Autodesk Inventor part; units mm, degrees
ref_plane "Work Plane2" through (11.25, 70.4, 1) normal (0, 1, 0) x (0, 0, 1)
ref_plane "Work Plane3" through (11.25, 42.7, 1) normal (0, -1, 0) x (1, 0, 0)
ref_plane "Work Plane4" through (11.925, 37.7, 1.675) normal (0, -1, 0) x (1, 0, 0)
ref_plane "Work Plane1" through (25.625, 84.2, 15.375) normal (0, 1, 0) x (0, 0, -1)
sketch "Sketch1" plane through (25.625, 84.2, 15.375) normal (0, 1, 0) x (0, 0, -1)
  line L0 (11.5, -1.5) -> (11, -1.5)
  line L1 (11, -1.5) -> (11, 1.5)
  line L2 (11, 1.5) -> (11.5, 1.5)
  line L3 (11.5, 1.5) -> (11.5, -1.5)
  line L4 (-12, -1.5) -> (-12, 1.5)
  line L5 (-12, 1.5) -> (-11.5, 1.5)
  line L6 (-11.5, 1.5) -> (-11.5, -1.5)
  line L7 (-11.5, -1.5) -> (-12, -1.5)
  circle A0 centre (0, 0) radius 5
  circle A1 centre (0, 0) radius 13.7
  line L8 (18.875, -15.375) -> (18.875, 116.625)
  line L9 (18.875, 116.625) -> (15.375, 116.625)
  line L10 (15.375, -15.375) -> (15.375, 116.625)
  line L11 (18.875, -15.375) -> (15.375, -15.375)
  line L12 (15.375, -15.375) -> (0, -15.375)
  line L13 (0, -15.375) -> (0, 15.375)
  line L14 (0, 15.375) -> (15.375, 15.375)
  line L15 (15.375, 15.375) -> (15.375, -15.375)
  circle A2 centre (12.125, 12.125) radius 3.25
  circle A3 centre (12.125, -12.125) radius 3.25
  line L16 (8.875, 15.375) -> (8.875, 10.4367)
  point P0 (15.375, 25.625)
  point P1 (0, -13.7)
  dimension "d2" = 15.375
  dimension "d3" = 15.375
  dimension "d4" = 6.5
  dimension "d5" = 6.5
ref_plane "Work Plane2" through (11.25, 70.4, 1) normal (0, 1, 0) x (0, 0, 1)
extrude "Extrusion1" add sketch "Sketch1" along normal blind 4 and the other way blind 13.8 contours A1 L16 A2 L10 A3 L12 L13 | L16 L14 A2 | A2 | A3 L10 L12 | A3 | L14 L10 A2
sketch "Sketch2" plane through (25.625, 70.4, 15.375) normal (0, -1, 0) x (1, 0, 0)
  arc A0 (-3.651, 5.9062) -> (-4.7619, 7.7035) centre (-4.2064, 6.8048) ccw
  arc A1 (-3.651, 5.9062) -> (-6.4477, 2.5768) centre (0, 0) ccw
  arc A2 (-8.4097, 3.3608) -> (-6.4477, 2.5768) centre (-7.4287, 2.9688) ccw
  arc A3 (-4.7619, 7.7035) -> (-8.4097, 3.3608) centre (0, 0) ccw
  arc A4 (6.4477, 2.5768) -> (8.4097, 3.3608) centre (7.4287, 2.9688) ccw
  arc A5 (6.4477, 2.5768) -> (3.651, 5.9062) centre (0, 0) ccw
  arc A6 (4.7619, 7.7035) -> (3.651, 5.9062) centre (4.2064, 6.8048) ccw
  arc A7 (8.4097, 3.3608) -> (4.7619, 7.7035) centre (0, 0) ccw
  arc A8 (-6.4563, -2.5553) -> (-8.4209, -3.3328) centre (-7.4386, -2.9441) ccw
  arc A9 (-6.4563, -2.5553) -> (-3.651, -5.9062) centre (0, 0) ccw
  arc A10 (-4.7619, -7.7035) -> (-3.651, -5.9062) centre (-4.2064, -6.8048) ccw
  arc A11 (-8.4209, -3.3328) -> (-4.7619, -7.7035) centre (0, 0) ccw
  arc A12 (3.651, -5.9062) -> (4.7619, -7.7035) centre (4.2064, -6.8048) ccw
  arc A13 (3.651, -5.9062) -> (6.4563, -2.5553) centre (0, 0) ccw
  arc A14 (8.4209, -3.3328) -> (6.4563, -2.5553) centre (7.4386, -2.9441) ccw
  arc A15 (4.7619, -7.7035) -> (8.4209, -3.3328) centre (0, 0) ccw
  circle A16 centre (10.65, 0.0124) radius 1.15
  circle A17 centre (0, 8) radius 1.0564
  circle A18 centre (0, -8) radius 1.0564
  circle A19 centre (0, 0) radius 5
  circle A20 centre (0, 0) radius 13.7
  line L0 (15.375, -18.875) -> (-116.625, -18.875)
  line L1 (-116.625, -18.875) -> (-116.625, -15.375)
  line L2 (15.375, -15.375) -> (-116.625, -15.375)
  line L3 (15.375, -18.875) -> (15.375, -15.375)
  line L4 (15.375, -15.375) -> (-15.375, -15.375)
  line L5 (-15.375, -15.375) -> (-15.375, 0)
  line L6 (-15.375, 0) -> (15.375, 0)
  line L7 (15.375, 0) -> (15.375, -15.375)
  circle A21 centre (0, 0) radius 14.375
  point P0 (-25.625, -15.375)
  point P1 (13.7, 0)
  point P2 (-13.7, 0)
  point P3 (-15.375, -15.375)
  point P4 (14.375, 0)
  point P5 (-14.375, 0)
  dimension "d10" = 15.375
  dimension "d11" = 15.375
ref_plane "Work Plane3" through (11.25, 42.7, 1) normal (0, -1, 0) x (1, 0, 0)
extrude "Extrusion2" add sketch "Sketch2" along normal up to surface (27.7 mm away) contours L6 L7 L2 L5 A21
sketch "Sketch3" plane through (25.625, 42.7, 15.375) normal (0, -1, 0) x (1, 0, 0)
  arc A0 (-3.651, 5.9062) -> (-4.7619, 7.7035) centre (-4.2064, 6.8048) ccw
  arc A1 (-3.651, 5.9062) -> (-6.4477, 2.5768) centre (0, 0) ccw
  arc A2 (-8.4097, 3.3608) -> (-6.4477, 2.5768) centre (-7.4287, 2.9688) ccw
  arc A3 (-4.7619, 7.7035) -> (-8.4097, 3.3608) centre (0, 0) ccw
  arc A4 (6.4477, 2.5768) -> (8.4097, 3.3608) centre (7.4287, 2.9688) ccw
  arc A5 (6.4477, 2.5768) -> (3.651, 5.9062) centre (0, 0) ccw
  arc A6 (4.7619, 7.7035) -> (3.651, 5.9062) centre (4.2064, 6.8048) ccw
  arc A7 (8.4097, 3.3608) -> (4.7619, 7.7035) centre (0, 0) ccw
  arc A8 (-6.4563, -2.5553) -> (-8.4209, -3.3328) centre (-7.4386, -2.9441) ccw
  arc A9 (-6.4563, -2.5553) -> (-3.651, -5.9062) centre (0, 0) ccw
  arc A10 (-4.7619, -7.7035) -> (-3.651, -5.9062) centre (-4.2064, -6.8048) ccw
  arc A11 (-8.4209, -3.3328) -> (-4.7619, -7.7035) centre (0, 0) ccw
  arc A12 (3.651, -5.9062) -> (4.7619, -7.7035) centre (4.2064, -6.8048) ccw
  arc A13 (3.651, -5.9062) -> (6.4563, -2.5553) centre (0, 0) ccw
  arc A14 (8.4209, -3.3328) -> (6.4563, -2.5553) centre (7.4386, -2.9441) ccw
  arc A15 (4.7619, -7.7035) -> (8.4209, -3.3328) centre (0, 0) ccw
  circle A16 centre (10.65, 0.0124) radius 1.15
  circle A17 centre (0, 8) radius 1.0564
  circle A18 centre (0, -8) radius 1.0564
  circle A19 centre (0, 0) radius 5
  circle A20 centre (0, 0) radius 13.7
  line L0 (15.375, -18.875) -> (-116.625, -18.875)
  line L1 (-116.625, -18.875) -> (-116.625, -15.375)
  line L2 (15.375, -15.375) -> (-116.625, -15.375)
  line L3 (15.375, -18.875) -> (15.375, -15.375)
  line L4 (15.375, 0) -> (15.375, -15.375)
  line L5 (15.375, -15.375) -> (-15.375, -15.375)
  line L6 (-15.375, -15.375) -> (-15.375, 0)
  line L7 (-15.375, 0) -> (15.375, 0)
  line L8 (15.375, 0) -> (15.375, -15.375)
  point P0 (-25.625, -15.375)
  point P1 (15.375, 0)
  point P2 (13.7, 0)
  point P3 (-13.7, 0)
  point P4 (-15.375, -15.375)
  dimension "d14" = 15.375
  dimension "d15" = 15.375
ref_plane "Work Plane4" through (11.925, 37.7, 1.675) normal (0, -1, 0) x (1, 0, 0)
extrude "Extrusion3" add sketch "Sketch3" along normal up to surface (5 mm away) contours L7 L4 L2 L6 A20
sketch "Sketch4" plane through (25.625, 37.7, 15.375) normal (0, -1, 0) x (1, 0, 0)
  circle A0 centre (-12.125, -12.125) radius 1.8
  circle A1 centre (12.125, -12.125) radius 1.8
  point P0 (-25.625, -15.375)
hole "Hole1" at (13.5, 37.7, 3.25) at (37.75, 37.7, 3.25) direction (0, 1, 0) diameter 4 depth 4.6 counterbore diameter 4.6 counterbore depth 0.6
sketch "Sketch5" plane through (25.625, 88.2, 15.375) normal (0, 1, 0) x (1, 0, 0)
  arc A0 (13.7, 0) -> (-10.4367, 8.875) centre (0, 0) ccw
  line L0 (13.7, 0) -> (15.375, 0)
  line L1 (15.375, 0) -> (15.375, 15.375)
  line L2 (15.375, 15.375) -> (-15.375, 15.375)
  line L3 (-15.375, 15.375) -> (-15.375, 8.875)
  line L4 (-15.375, 8.875) -> (-10.4367, 8.875)
  circle A1 centre (12.125, 12.125) radius 3.25
  circle A2 centre (-12.125, 12.125) radius 3.25
  point P0 (-25.625, 15.375)
  dimension "d25" = 6.5
  dimension "d26" = 6.5
hole "Hole2" at (37.75, 88.2, 3.25) at (13.5, 88.2, 3.25) direction (0, -1, 0) diameter 4 depth 9 counterbore diameter 5 counterbore depth 1
equation "\"d3\" = d2"
equation "\"d11\" = d10"
equation "\"d15\" = d14"
properties part number "motur_holder"
Could you check a few things on this model? Use its own coordinates, in mm. A direction names the side the tool comes from. Round coordinates to 2 decimals unless told otherwise and drop trailing zeros. Write each loop counter-clockwise with the first axis right and the second up, starting at its lowest first coordinate (ties: lowest second). Pieces come first, ordered by that corner, then holes. Notation, with made-up numbers: (-16.5, 1.5) -> (16.5, 1.5) arc R14 cw to (16.5, 5.5) -> close; hole circle Ø8 at (-19.5, 80.5). An arc over 180 degrees is marked (long way). Use a Markdown table: item, result.
1. Which directions (+Z, -Z, +X, -X, +Y, -Y) give clear straight access to the entire face, cutting with the end or side of a thin tool? Please do faces 1 (the face through (39.79, 38, 2.19)), 2 (the face through (36, 87.2, 2)), 3 (the face through (13, 79, 6.5)).
Answer key:
| item | result |
|---|---|
| face 1 | -Y |
| face 2 | +Y |
| face 3 | +Z, -X, +Y |
2. If we section it at A-A (z = 14.75): List the corners of the cut face in (x, y) for me, then the cut area to 3 significant figures.
Answer key:
| item | result |
|---|---|
| outline | (10.25, 37.7) -> (11.94, 37.7) -> (11.94, 42.7) -> (11.26, 42.7) -> (11.26, 70.4) -> (10.25, 70.4) -> close; (39.31, 37.7) -> (41, 37.7) -> (41, 88.2) -> (39.31, 88.2) -> (39.31, 70.4) -> (39.99, 70.4) -> (39.99, 42.7) -> (39.31, 42.7) -> close |
| area | 103 mm^2 |
3. For pin 1 Ø1.5 at (x, y) = (20, 50) entering from +Z; pin 2 Ø3 at (x, z) = (37.75, 3.25) entering from +Y; pin 3 Ø4.5 at (x, z) = (13.5, 3.25) entering from +Y, each with a flat end and sliding along its axis, tell me the tip position at first contact or that it passes through.
Answer key:
| item | result |
|---|---|
| pin 1 | stops at z = 2.49 |
| pin 2 | stops at y = 79.2 |
| pin 3 | stops at y = 87.2 |
4. We'd pull the mould along Y, two halves only. Please class faces 4 (the face through (11.22, 38, 3.55)), 5 (the face through (27, 37.7, 1)), 6 (the face through (25.6, 42.7, 1.3)), 7 (the face through (14, 87.2, 1)): +Y half, -Y half, draft (parallel to the pull), parting line (faces both ways), or undercut.
Answer key:
| item | result |
|---|---|
| face 4 | draft |
| face 5 | -Y half |
| face 6 | undercut |
| face 7 | +Y half |
5. If we section it at D-D (z = 12.5): List the corners of the cut face in (x, y) for me.
Answer key:
| item | result |
|---|---|
| outline | (10.25, 37.7) -> (12.23, 37.7) -> (12.23, 42.7) -> (11.54, 42.7) -> (11.54, 70.4) -> (10.25, 70.4) -> close; (39.02, 37.7) -> (41, 37.7) -> (41, 88.2) -> (39.02, 88.2) -> (39.02, 70.4) -> (39.71, 70.4) -> (39.71, 42.7) -> (39.02, 42.7) -> close |
6. If we section it at B-B (y = 74): List the corners of the cut face in (x, z) for me (3 decimals), then the cut area to 3 significant figures.
Answer key:
| item | result |
|---|---|
| outline | (10.25, 0) -> (41, 0) -> (41, 15.375) -> (39.325, 15.375) arc R13.7 cw to (15.188, 6.5) -> (10.25, 6.5) -> close |
| area | 154 mm^2 |
7. Please list where these lines run through material, in increasing order: probe 1 along X at (y, z) = (81.75, 3.25); probe 2 along X at (y, z) = (87.6, 3.25); probe 3 along Y at (x, z) = (36, 5.5).
Answer key:
| item | result |
|---|---|
| probe 1 | x = 10.25 to 11.5, 15.5 to 19.25, 32 to 35.75, 39.75 to 41 |
| probe 2 | x = 10.25 to 11, 16 to 19.25, 32 to 35.25, 40.25 to 41 |
| probe 3 | y = 37.7 to 42.7, 70.4 to 88.2 |
8. If we section it at C-C (x = 16.5): List the corners of the cut face in (y, z) for me.
Answer key:
| item | result |
|---|---|
| outline | (37.7, 0) -> (88.2, 0) -> (88.2, 5.16) -> (70.4, 5.16) -> (70.4, 4.27) -> (42.7, 4.27) -> (42.7, 5.16) -> (37.7, 5.16) -> close |
